For this review, take the finished solid that the model builds, in its own axes (mm). Face numbers are marked on the shaded views. A direction names the side the tool comes from. Give positions to 0.01 mm unless a question says otherwise; leave off trailing zeros. Loops run counter-clockwise (first coordinate to the right, second up) from the corner with the lowest first, then second, coordinate; pieces in that order, holes last. Notation, with made-up numbers: (24.25, 59) - (33.25, 59) arc R11 ccw to (33.25, 73) - close; hole circle Ø7 at (-39.5, 4). An arc over 180 degrees is marked (long way). Answer as CSV lines item,"result".
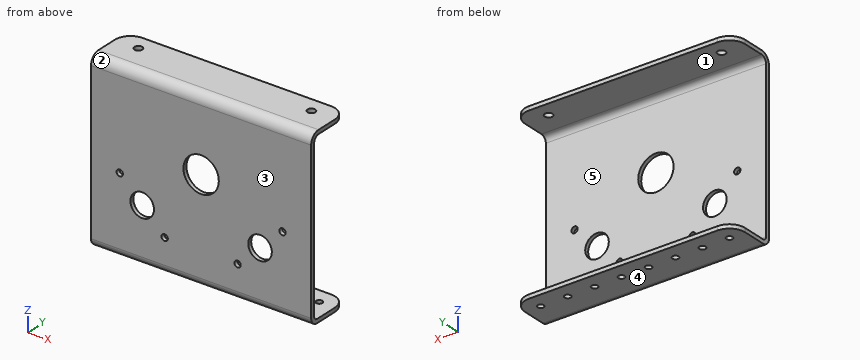
from build123d import *

# Parameters (mm, degrees)
SKETCH1_W           = 177.8
SKETCH1_H           = 127
BOSS_EXTRUDE1_DEPTH = 3.175
EDGE_FLANGE1_DEPTH  = 177.8
EDGE_FLANGE2_DEPTH  = 177.8
SKETCH17_R          = 2.54
CUT_EXTRUDE1_DEPTH  = 5.08
FILLET1_R           = 12.7
SKETCH18_R          = 3.175
CUT_EXTRUDE2_DEPTH  = 5.08
SKETCH19_R          = 14.2875
CUT_EXTRUDE3_DEPTH  = 12.7
SKETCH20_R          = 9.525
CUT_EXTRUDE4_DEPTH  = 12.7
SKETCH21_R          = 2.54
CUT_EXTRUDE6_DEPTH  = 12.7


# Sheet-metal steps are written as plain solids
with BuildPart() as part:
    # Sketch1 → Boss-Extrude1 (new body)
    with BuildSketch(Plane(origin=(0, 0, 0), x_dir=(1, 0, 0), z_dir=(0, 1, 0))):
        Rectangle(SKETCH1_W, SKETCH1_H)
    extrude(amount=BOSS_EXTRUDE1_DEPTH)

    # Edge-Flange1 section (across the edge) → Edge-Flange1 (add)
    with BuildSketch(Plane(origin=(88.9, 3.175, -66.675), x_dir=(0, 0, 1), z_dir=(-1, 0, 0))):
        with BuildLine():
            Line((-3.175, 3.175), (-3.175, 34.925))
            Line((-3.175, 34.925), (0, 34.925))
            Line((0, 34.925), (0, 3.175))
            ThreePointArc((0, 3.175), (0.92993597, 0.92993597), (3.175, 0))
            Line((3.175, 0), (3.175, -3.175))
            ThreePointArc((3.175, -3.175), (-1.315128061, -1.315128061), (-3.175, 3.175))
        make_face()
    extrude(amount=EDGE_FLANGE1_DEPTH)

    # Edge-Flange2 section (across the edge) → Edge-Flange2 (add)
    with BuildSketch(Plane(origin=(-88.9, 3.175, 68.199), x_dir=(0, 0, -1), z_dir=(1, 0, 0))):
        with BuildLine():
            Line((-3.175, 4.699), (-3.175, 34.925))
            Line((-3.175, 34.925), (0, 34.925))
            Line((0, 34.925), (0, 4.699))
            ThreePointArc((0, 4.699), (1.376305235, 1.376305235), (4.699, 0))
            Line((4.699, 0), (4.699, -3.175))
            ThreePointArc((4.699, -3.175), (-0.868758795, -0.868758795), (-3.175, 4.699))
        make_face()
    extrude(amount=EDGE_FLANGE2_DEPTH)

    # Sketch17 → Cut-Extrude1 (cut)
    with BuildSketch(Plane(origin=(0, 0, -69.85), x_dir=(-1, 0, 0), z_dir=(0, 0, -1))):
        with Locations(Location((-76.2, 25.4, 0), (0, 0, 90))):
            Circle(SKETCH17_R)
        with Locations(Location((-54.428571429, 25.4, 0), (0, 0, 90))):
            Circle(SKETCH17_R)
        with Locations(Location((-32.657142857, 25.4, 0), (0, 0, 90))):
            Circle(SKETCH17_R)
        with Locations(Location((-10.885714286, 25.4, 0), (0, 0, 90))):
            Circle(SKETCH17_R)
        with Locations(Location((10.885714286, 25.4, 0), (0, 0, 90))):
            Circle(SKETCH17_R)
        with Locations(Location((32.657142857, 25.4, 0), (0, 0, 90))):
            Circle(SKETCH17_R)
        with Locations(Location((54.428571429, 25.4, 0), (0, 0, 90))):
            Circle(SKETCH17_R)
        with Locations(Location((76.2, 25.4, 0), (0, 0, 90))):
            Circle(SKETCH17_R)
    extrude(amount=-CUT_EXTRUDE1_DEPTH, mode=Mode.SUBTRACT)

    # Fillet1
    fillet1_edges = [part.edges().sort_by_distance(p)[0] for p in [
        (88.9, 38.1, -68.2625),
        (-88.9, 38.1, -68.2625),
        (-88.9, 38.1, 69.7865),
        (88.9, 38.1, 69.7865),
    ]]
    fillet(fillet1_edges, radius=FILLET1_R)

    # Sketch18 → Cut-Extrude2 (cut)
    with BuildSketch(Plane(origin=(0, 0, 68.199), x_dir=(-1, 0, 0), z_dir=(0, 0, -1))):
        with Locations((69.85, 25.4)):
            Circle(SKETCH18_R)
        with Locations((-69.85, 25.4)):
            Circle(SKETCH18_R)
    extrude(amount=-CUT_EXTRUDE2_DEPTH, mode=Mode.SUBTRACT)

    # Sketch19 → Cut-Extrude3 (cut)
    with BuildSketch(Plane(origin=(0, 0, 0), x_dir=(-1, 0, 0), z_dir=(0, -1, 0))):
        with Locations(Location((0, -12.7, 0), (0, 0, 90))):
            Circle(SKETCH19_R)
    extrude(amount=-CUT_EXTRUDE3_DEPTH, mode=Mode.SUBTRACT)

    # Sketch20 → Cut-Extrude4 (cut)
    with BuildSketch(Plane.XZ):
        with Locations(Location((47.586884748, -25.4, 0), (0, 0, 270))):
            Circle(SKETCH20_R)
        with Locations(Location((-47.586884748, -25.4, 0), (0, 0, 270))):
            Circle(SKETCH20_R)
    extrude(amount=-CUT_EXTRUDE4_DEPTH, mode=Mode.SUBTRACT)

    # Sketch21 → Cut-Extrude6 (cut)
    with BuildSketch(Plane(origin=(0, 0, 0), x_dir=(-1, 0, 0), z_dir=(0, -1, 0))):
        with Locations(Location((-65.726112956, 7.62, 0), (0, 0, 90))):
            Circle(SKETCH21_R)
        with Locations(Location((-29.447656539, 43.18, 0), (0, 0, 90))):
            Circle(SKETCH21_R)
        with Locations(Location((65.726112956, 7.62, 0), (0, 0, 90))):
            Circle(SKETCH21_R)
        with Locations(Location((29.447656539, 43.18, 0), (0, 0, 90))):
            Circle(SKETCH21_R)
    extrude(amount=-CUT_EXTRUDE6_DEPTH, mode=Mode.SUBTRACT)


solid = part.part
1) Draft analysis for pull direction Z (two halves, no side actions). For the marked faces 1, 2 and 3, state which applies: pulls with the +Z half, pulls with the -Z half, needs draft (parallel to the pull), parting line crosses it, or undercut.
From the geometry:
face 1,"undercut"
face 2,"pulls with the +Z half"
face 3,"needs draft"
2) Machinability: for the marked faces 4 and 5, which of the approach directions +Z, -Z, +X, -X, +Y, -Y give a long, thin tool a straight path to every point of the face, cutting with its end or side? Answer none if there is none.
From the geometry:
face 4,"-Z, +X, -X, +Y, -Y"
face 5,"+X, -X, +Y"
3) Insertion check: P1, Ø3, axis at x = 10.89, y = 25.4, coming from the -Z side; P2, Ø2, axis at x = 62, z = 0.5, coming from the +Y side (3 decimals). Each pin has a flat end and moves straight along its axis. Give the tip position at first contact, or say it passes through.
From the geometry:
P1,"stops at z = 68.2"
P2,"stops at y = 3.175"
4) Consider section D-D on z = -43.18. Write out the cut boundary in (x, y) (3 decimals).
From the geometry:
outline,"(-88.9, 0) - (-31.988, 0) - (-31.988, 3.175) - (-88.9, 3.175) - close; (-26.908, 0) - (26.908, 0) - (26.908, 3.175) - (-26.908, 3.175) - close; (31.988, 0) - (88.9, 0) - (88.9, 3.175) - (31.988, 3.175) - close"
5) Consider section A-A on z = 12.7. Write out the cut boundary in (x, y) (1 decimal).
From the geometry:
outline,"(-88.9, 0) - (-14.3, 0) - (-14.3, 3.2) - (-88.9, 3.2) - close; (14.3, 0) - (88.9, 0) - (88.9, 3.2) - (14.3, 3.2) - close"
6) Wall thickness on line 1 (Z direction, x = -59.5, y = 36.5) (3 decimals); line 2 (Y direction, x = 69.85, z = 69.8) (3 decimals); line 3 (Y direction, x = 26, z = 38) (3 decimals): over which ranges is each line inside the solid? List them lowest first. Write a range as from..to.
From the geometry:
line 1,"z = -69.85..-66.675, 68.199..71.374"
line 2,"y = 3.151..22.225, 28.575..38.1"
line 3,"y = 0..3.175"
7) Consider section C-C on y = 12. Write out the cut boundary in (x, z) (3 decimals).
From the geometry:
outline,"(-88.9, -69.85) - (88.9, -69.85) - (88.9, -66.675) - (-88.9, -66.675) - close; (-88.9, 68.199) - (88.9, 68.199) - (88.9, 71.374) - (-88.9, 71.374) - close"
